CAD build for the part. Positions are in the model's coordinates, mm. Coordinates: 2 decimals unless noted, no trailing zeros. Loops run counter-clockwise (first coordinate to the right, second up) from the corner with the lowest first, then second, coordinate; pieces in that order, holes last.
1) Two-plate mould, pull along Y, no slides. Class faces 1 (the flat face through (0, 0, 135)), 2 (the cylindrical face through (-0.06, 0.07, 13.5)), 3 (the cylindrical face through (4.16, -1.72, 66.55)): +Y half, -Y half, draft (parallel to the pull), parting line (faces both ways), or undercut.
2) Saw through at D-D, the plane z = 12. Write the cut outline in (x, y).
3) Saw through at A-A, the plane y = 0. Write the cut outline in (x, z), and give its area (3 significant figures).
4) Wall check: line 1 along Z through (x, y) = (0.5, 0); line 2 along Y through (x, z) = (-2.25, 12); line 3 along Y through (x, z) = (0.25, 12). Give the ranges that are in metal, low to high.
5) Saw through at C-C, the plane z = 58. Write the cut outline in (x, y), and give its area (3 significant figures).
6) Saw through at B-B, the plane x = 1. Write the cut outline in (y, z).
7) Pin check, flat tips, straight feed: pin 1 Ø4 at (y, z) = (0, 12) entering from -X; pin 2 Ø4 at (y, z) = (3, 106) entering from +X; pin 3 Ø4 at (x, z) = (-3, 72) entering from +Y; pin 4 Ø4 at (y, z) = (3.5, 79) entering from +X. Stop position of each tip, or through.
```python
from build123d import *

# Parameters (mm, degrees)
IZIM1_R                                = 4.5
Y_KSEKLIK_EKSTR_ZYON1_DEPTH            = 15
KES_EKSTR_ZYON1_REACH                  = 18.294
KES_EKSTR_ZYON1_END_RADIUS             = 4.5
IZIM2_R                                = 1.5
KES_EKSTR_ZYON1_DIRECTION_2_REACH      = 18.294
KES_EKSTR_ZYON1_DIRECTION_2_END_RADIUS = 4.5
IZIM3_R                                = 4.5
Y_KSEKLIK_EKSTR_ZYON2_DEPTH            = 120


with BuildPart() as part:
    # Çizim1 → Yükseklik-Ekstrüzyon1 (new body)
    with BuildSketch(Plane.XY):
        Circle(IZIM1_R)
    extrude(amount=Y_KSEKLIK_EKSTR_ZYON1_DEPTH)

    # Kes-Ekstrüzyon1: up to this cylinder (the profile starts inside it)
    kes_ekstr_zyon1_end = Plane(origin=(0, 0, 12), z_dir=(0, 0, -1)) * Cylinder(KES_EKSTR_ZYON1_END_RADIUS, 46.588, mode=Mode.PRIVATE)
    # Çizim2 → Kes-Ekstrüzyon1 (cut, up to the surface)
    with BuildSketch(Plane(origin=(0, 0, 0), x_dir=(0, 0, -1), z_dir=(1, 0, 0)), mode=Mode.PRIVATE) as kes_ekstr_zyon1_sk1:
        with Locations((-12, 0)):
            Circle(IZIM2_R)
    kes_ekstr_zyon1_tool1 = extrude(kes_ekstr_zyon1_sk1.sketch, amount=-KES_EKSTR_ZYON1_REACH, mode=Mode.PRIVATE) & kes_ekstr_zyon1_end
    add(kes_ekstr_zyon1_tool1.solids().sort_by_distance((0, 0, 12))[0], mode=Mode.SUBTRACT)

    # Kes-Ekstrüzyon1 direction 2: up to this cylinder (the profile starts inside it)
    kes_ekstr_zyon1_direction_2_end = Plane(origin=(0, 0, 12), z_dir=(0, 0, -1)) * Cylinder(KES_EKSTR_ZYON1_DIRECTION_2_END_RADIUS, 46.588, mode=Mode.PRIVATE)
    # Çizim2 → Kes-Ekstrüzyon1 direction 2 (cut, up to the surface)
    with BuildSketch(Plane(origin=(0, 0, 0), x_dir=(0, 0, -1), z_dir=(1, 0, 0)), mode=Mode.PRIVATE) as kes_ekstr_zyon1_direction_2_sk1:
        with Locations((-12, 0)):
            Circle(IZIM2_R)
    kes_ekstr_zyon1_direction_2_tool1 = extrude(kes_ekstr_zyon1_direction_2_sk1.sketch, amount=KES_EKSTR_ZYON1_DIRECTION_2_REACH, mode=Mode.PRIVATE) & kes_ekstr_zyon1_direction_2_end
    add(kes_ekstr_zyon1_direction_2_tool1.solids().sort_by_distance((0, 0, 12))[0], mode=Mode.SUBTRACT)

    # Çizim3 → Yükseklik-Ekstrüzyon2 (add)
    with BuildSketch(Plane.XY.offset(15)):
        Circle(IZIM3_R)
    extrude(amount=Y_KSEKLIK_EKSTR_ZYON2_DEPTH)


solid = part.part
```
Data:
1. face 1: draft
1. face 2: undercut
1. face 3: parting line
2. outline: (-4.24, -1.5) arc R4.5 ccw to (4.24, -1.5) - close; (-4.24, 1.5) - (4.24, 1.5) arc R4.5 ccw to start
3. outline: (-4.5, 0) - (4.5, 0) - (4.5, 10.5) - (-4.5, 10.5) - close; (-4.5, 13.5) - (4.5, 13.5) - (4.5, 135) - (-4.5, 135) - close
3. area: 1,190 mm2
4. line 1: z = 0 to 10.5, 13.5 to 135
4. line 2: y = -3.9 to -1.5, 1.5 to 3.9
4. line 3: y = -4.49 to -1.5, 1.5 to 4.49
5. outline: circle Ø9 at (0, 0)
5. area: 63.6 mm2
6. outline: (-4.39, 0) - (4.39, 0) - (4.39, 135) - (-4.39, 135) - close; hole circle Ø3 at (0, 12)
7. pin 1: stops at x = -4.5
7. pin 2: stops at x = 4.39
7. pin 3: stops at y = 4.39
7. pin 4: stops at x = 4.24
